from build123d import *

# Parameters (mm, degrees)
SKETCH1_R                                       = 1.5
BOSS_EXTRUDE1_DEPTH                             = 2
BOSS_EXTRUDE2_DEPTH                             = 2
BOSS_EXTRUDE3_DEPTH                             = 13.5
CSK_FOR_M3_FLAT_HEAD_MACHINE_SCREW1_D           = 3.4
CSK_FOR_M3_FLAT_HEAD_MACHINE_SCREW1_CSINK_D     = 6.5
CSK_FOR_M3_FLAT_HEAD_MACHINE_SCREW1_CSINK_ANGLE = 90


with BuildPart() as part:
    # Sketch1 → Boss-Extrude1 (new body)
    with BuildSketch(Plane.XY):
        with BuildLine():
            Line((-21.64147317, 1.655195806), (-14.910368292, 16.463798951))
            ThreePointArc((-14.910368292, 16.463798951), (-14.541387592, 16.890773142), (-14, 17.05))
            Line((-14, 17.05), (14, 17.05))
            ThreePointArc((14, 17.05), (14.541387592, 16.890773142), (14.910368292, 16.463798951))
            Line((14.910368292, 16.463798951), (21.64147317, 1.655195806))
            ThreePointArc((21.64147317, 1.655195806), (22, 0), (21.64147317, -1.655195806))
            Line((21.64147317, -1.655195806), (14.910368292, -16.463798951))
            ThreePointArc((14.910368292, -16.463798951), (14.541387592, -16.890773142), (14, -17.05))
            Line((14, -17.05), (-14, -17.05))
            ThreePointArc((-14, -17.05), (-14.541387592, -16.890773142), (-14.910368292, -16.463798951))
            Line((-14.910368292, -16.463798951), (-21.64147317, -1.655195806))
            ThreePointArc((-21.64147317, -1.655195806), (-22, 0), (-21.64147317, 1.655195806))
        make_face()
        with Locations((-18, 0)):
            Circle(SKETCH1_R, mode=Mode.SUBTRACT)
        with Locations((18, 0)):
            Circle(SKETCH1_R, mode=Mode.SUBTRACT)
    extrude(amount=BOSS_EXTRUDE1_DEPTH)

    # Sketch2 → Boss-Extrude2 (add)
    with BuildSketch(Plane.XY.offset(2)):
        with BuildLine():
            Line((-12, 16), (12, 16))
            ThreePointArc((12, 16), (13.414213562, 15.414213562), (14, 14))
            Line((14, 14), (14, -14))
            ThreePointArc((14, -14), (13.414213562, -15.414213562), (12, -16))
            Line((12, -16), (-12, -16))
            ThreePointArc((-12, -16), (-13.414213562, -15.414213562), (-14, -14))
            Line((-14, -14), (-14, 14))
            ThreePointArc((-14, 14), (-13.414213562, 15.414213562), (-12, 16))
        make_face()
    extrude(amount=BOSS_EXTRUDE2_DEPTH)

    # Sketch3 → Boss-Extrude3 (add, symmetric)
    with BuildSketch(Plane(origin=(0, 0, 0), x_dir=(0, 0, -1), z_dir=(1, 0, 0))):
        Polygon((0, 15.5), (13.171636249, 15.5), (13.171636249, 0), (40, 0), (40, -15.5), (0, -15.5), align=None)
    extrude(amount=BOSS_EXTRUDE3_DEPTH, both=True)

    # CSK for M3 Flat Head Machine Screw1 (through all)
    with Locations(Plane.XY.offset(2)):
        with Locations((-18, 0), (18, 0)):
            CounterSinkHole(CSK_FOR_M3_FLAT_HEAD_MACHINE_SCREW1_D / 2, CSK_FOR_M3_FLAT_HEAD_MACHINE_SCREW1_CSINK_D / 2, counter_sink_angle=CSK_FOR_M3_FLAT_HEAD_MACHINE_SCREW1_CSINK_ANGLE)


solid = part.part
Geometry check sheet. Reference: the model listing, model coordinates, mm. A direction names the side the tool comes from. Coordinates: 2 decimals unless noted, no trailing zeros. Order: outer loops, then holes, each group sorted by start corner. A loop starts at its lowest first (then second) coordinate and runs counter-clockwise, first axis right, second up. Notation, with made-up numbers: (64.5, 84.25) - (78.5, 84.25) arc R26 cw to (78.5, 109.25) - close; hole circle Ø6 at (41, 38). An arc over 180 degrees is marked (long way). Answer in a Markdown table with one row per item. Add a question column.
1) Material ranges on line 1 along X through (y, z) = (0, 0.1); line 2 along Y through (x, z) = (2, -30.5); line 3 along Z through (x, y) = (-17, -5), recorded low to high. Write a range as [from, to].
2) Cross-section at B-B, the plane x = -18. Record the cut outline in (y, z), then the cut area to 3 significant figures.
3) Cross-section at A-A, the plane x = 5. Record the cut outline in (y, z).
4) Cross-section at C-C, the plane z = -36. Record the cut outline in (x, y), then the cut area to 4 significant figures.
5) Gauge pin test, flat ends, axial feed: P1, Ø8, axis at x = 3, z = -18.5, coming from the -Y side; P2, Ø4.5, axis at x = 4.5, y = 8, coming from the -Z side; P3, Ø9.5, axis at y = -6, z = -13, coming from the +X side; P4, Ø12, axis at x = -0.5, y = 0.5, coming from the -Z side. Record the tip position at first contact, or that the pin passes through.
6) Cross-section at D-D, the plane y = -13. Record the cut outline in (x, z).
7) Set-up check for faces 1 (the cylindrical face through (13.43, -15.4, 2.99)), 2 (the flat face through (0, 15.5, -6)), 3 (the cylindrical face through (13.4, 15.43, 2.99)): record each of +Z, -Z, +X, -X, +Y, -Y from which the full face is reachable in a straight line by a thin tool's end or side.
Check result:
| question | item | result |
|---|---|---|
| 1 | line 1 | x = [-22, -19.7], [-16.3, 16.3], [19.7, 22] |
| 1 | line 2 | y = [-15.5, 0] |
| 1 | line 3 | z = [0, 2] |
| 2 | outline | (-9.67, 0) - (-1.7, 0) - (-1.7, 0.45) - (-3.25, 2) - (-9.67, 2) - close; (1.7, 0) - (9.67, 0) - (9.67, 2) - (3.25, 2) - (1.7, 0.45) - close |
| 2 | area | 29.5 mm² |
| 3 | outline | (-17.05, 0) - (-15.5, 0) - (-15.5, -40) - (0, -40) - (0, -13.17) - (15.5, -13.17) - (15.5, 0) - (17.05, 0) - (17.05, 2) - (16, 2) - (16, 4) - (-16, 4) - (-16, 2) - (-17.05, 2) - close |
| 4 | outline | (-13.5, -15.5) - (13.5, -15.5) - (13.5, 0) - (-13.5, 0) - close |
| 4 | area | 418.5 mm² |
| 5 | P1 | stops at y = -15.5 |
| 5 | P2 | stops at z = -13.17 |
| 5 | P3 | stops at x = 13.5 |
| 5 | P4 | stops at z = -40 |
| 6 | outline | (-16.48, 0) - (-13.5, 0) - (-13.5, -40) - (13.5, -40) - (13.5, 0) - (16.48, 0) - (16.48, 2) - (14, 2) - (14, 4) - (-14, 4) - (-14, 2) - (-16.48, 2) - close |
| 7 | face 1 | +Z, +X, -Y |
| 7 | face 2 | -Z, +X, -X, +Y |
| 7 | face 3 | +Z, +X, +Y |
